Print and shaded views of the part. All mm, measured from the part's lowest x, y and z. Coordinates: 2 decimals unless noted, no trailing zeros. Order: outer loops, then holes, each group sorted by start corner. A loop starts at its lowest first (then second) coordinate and runs counter-clockwise, first axis right, second up. Notation, with made-up numbers: M 6.5,-34 L 53.5,-34 A20 ccw 53.5,-9 Z; hole C 40,75 d11. An arc over 180 degrees is marked long. Return JSON: item names as keys, results as strings.
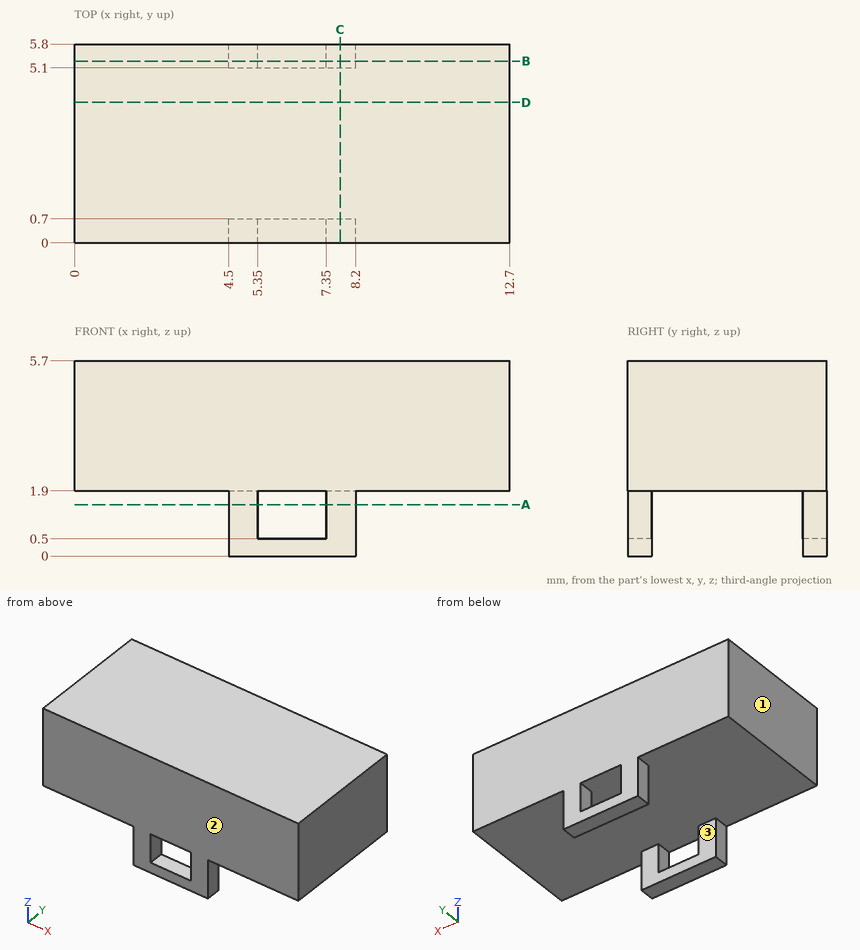
Item 1: Wall check: line 1 (X direction, y = 5.55, z = 1.7); line 2 (Z direction, x = 10, y = 1.95). Give the ranges that are in metal, low to high.
Check result:
{"line 1": "x = 4.5 to 5.35, 7.35 to 8.2", "line 2": "z = 1.9 to 5.7"}
Item 2: Saw through at A-A (z = 1.5). Write the cut outline in (x, y).
Check result:
{"outline": "M 4.5,0 L 5.35,0 L 5.35,0.7 L 4.5,0.7 Z; M 4.5,5.1 L 5.35,5.1 L 5.35,5.8 L 4.5,5.8 Z; M 7.35,0 L 8.2,0 L 8.2,0.7 L 7.35,0.7 Z; M 7.35,5.1 L 8.2,5.1 L 8.2,5.8 L 7.35,5.8 Z"}
Item 3: Saw through at D-D (y = 4.1). Write the cut outline in (x, z), and give its area (3 significant figures).
Check result:
{"outline": "M 0,1.9 L 12.7,1.9 L 12.7,5.7 L 0,5.7 Z", "area": "48.3 mm2"}
Item 4: Pull direction Y, two halves, no side cores. Call the marked faces 1, 2 and 3: +Y half, -Y half, draft (parallel to the pull), parting line (faces both ways), or undercut.
Check result:
{"face 1": "draft", "face 2": "-Y half", "face 3": "undercut"}
Item 5: Saw through at C-C (x = 7.75). Write the cut outline in (y, z), and give its area (3 significant figures).
Check result:
{"outline": "M 0,0 L 0.7,0 L 0.7,1.9 L 5.1,1.9 L 5.1,0 L 5.8,0 L 5.8,5.7 L 0,5.7 Z", "area": "24.7 mm2"}
Item 6: Saw through at B-B (y = 5.3). Write the cut outline in (x, z), and give its area (3 significant figures).
Check result:
{"outline": "M 0,1.9 L 4.5,1.9 L 4.5,0 L 8.2,0 L 8.2,1.9 L 12.7,1.9 L 12.7,5.7 L 0,5.7 Z; hole M 5.35,0.5 L 7.35,0.5 L 7.35,1.9 L 5.35,1.9 Z", "area": "52.5 mm2"}
Item 7: Drop flat-ended pins along their axis: pin 1 Ø0.6 at (y, z) = (5.5, 1.5) entering from -X; pin 2 Ø0.8 at (y, z) = (5.5, 1) entering from +X. Give the stop position or say it passes through.
Check result:
{"pin 1": "stops at x = 4.5", "pin 2": "stops at x = 8.2"}
